from build123d import *

# Parameters (mm, degrees)
SKETCH21_R          = 1.625
SKETCH21_R_2        = 7.5
MAIN_DEPTH          = 2
SKETCH23_R          = 4.2
SKETCH23_R_2        = 3.2
BOSS_EXTRUDE1_DEPTH = 2
REVOLVE1_START      = 2
REVOLVE1_DEPTH      = 3.0000001
REVOLVE1_2_ANGLE    = 20
REVOLVE1_3_ANGLE    = 20
CIRPATTERN1_COUNT   = 4


with BuildPart() as part:
    # Sketch21 → Main (new body)
    with BuildSketch(Plane(origin=(0, 0, 0), x_dir=(1, 0, 0), z_dir=(0, 1, 0))):
        with BuildLine():
            Line((-12.374368671, 10.960155108), (-10.960155108, 12.374368671))
            ThreePointArc((-10.960155108, 12.374368671), (-8.838834765, 13.253048327), (-6.717514421, 12.374368671))
            Line((-6.717514421, 12.374368671), (-6.969531846, 12.626386096))
            ThreePointArc((-6.969531846, 12.626386096), (-5.176380902, 11.591109915), (-3.105828541, 11.591109915))
            ThreePointArc((-3.105828541, 11.591109915), (0, 12), (3.105828541, 11.591109915))
            ThreePointArc((3.105828541, 11.591109915), (5.176380902, 11.591109915), (6.969531846, 12.626386096))
            Line((6.969531846, 12.626386096), (6.717514421, 12.374368671))
            ThreePointArc((6.717514421, 12.374368671), (8.838834765, 13.253048327), (10.960155108, 12.374368671))
            Line((10.960155108, 12.374368671), (12.374368671, 10.960155108))
            ThreePointArc((12.374368671, 10.960155108), (13.253048327, 8.838834765), (12.374368671, 6.717514421))
            Line((12.374368671, 6.717514421), (12.626386096, 6.969531846))
            ThreePointArc((12.626386096, 6.969531846), (11.591109915, 5.176380902), (11.591109915, 3.105828541))
            ThreePointArc((11.591109915, 3.105828541), (12, 0), (11.591109915, -3.105828541))
            ThreePointArc((11.591109915, -3.105828541), (11.591109915, -5.176380902), (12.626386096, -6.969531846))
            Line((12.626386096, -6.969531846), (12.374368671, -6.717514421))
            ThreePointArc((12.374368671, -6.717514421), (13.253048327, -8.838834765), (12.374368671, -10.960155108))
            Line((12.374368671, -10.960155108), (10.960155108, -12.374368671))
            ThreePointArc((10.960155108, -12.374368671), (8.838834765, -13.253048327), (6.717514421, -12.374368671))
            Line((6.717514421, -12.374368671), (6.969531846, -12.626386096))
            ThreePointArc((6.969531846, -12.626386096), (5.176380902, -11.591109915), (3.105828541, -11.591109915))
            ThreePointArc((3.105828541, -11.591109915), (0, -12), (-3.105828541, -11.591109915))
            ThreePointArc((-3.105828541, -11.591109915), (-5.176380902, -11.591109915), (-6.969531846, -12.626386096))
            Line((-6.969531846, -12.626386096), (-6.717514421, -12.374368671))
            ThreePointArc((-6.717514421, -12.374368671), (-8.838834765, -13.253048327), (-10.960155108, -12.374368671))
            Line((-10.960155108, -12.374368671), (-12.374368671, -10.960155108))
            ThreePointArc((-12.374368671, -10.960155108), (-13.253048327, -8.838834765), (-12.374368671, -6.717514421))
            Line((-12.374368671, -6.717514421), (-12.626386096, -6.969531846))
            ThreePointArc((-12.626386096, -6.969531846), (-11.591109915, -5.176380902), (-11.591109915, -3.105828541))
            ThreePointArc((-11.591109915, -3.105828541), (-12, 0), (-11.591109915, 3.105828541))
            ThreePointArc((-11.591109915, 3.105828541), (-11.591109915, 5.176380902), (-12.626386096, 6.969531846))
            Line((-12.626386096, 6.969531846), (-12.374368671, 6.717514421))
            ThreePointArc((-12.374368671, 6.717514421), (-13.253048327, 8.838834765), (-12.374368671, 10.960155108))
        make_face()
        with Locations(Location((8.838834765, 8.838834765, 0), (0, 0, 270))):
            Circle(SKETCH21_R, mode=Mode.SUBTRACT)
        with Locations(Location((8.838834765, -8.838834765, 0), (0, 0, 270))):
            Circle(SKETCH21_R, mode=Mode.SUBTRACT)
        with Locations(Location((-8.838834765, -8.838834765, 0), (0, 0, 270))):
            Circle(SKETCH21_R, mode=Mode.SUBTRACT)
        with Locations(Location((-8.838834765, 8.838834765, 0), (0, 0, 270))):
            Circle(SKETCH21_R, mode=Mode.SUBTRACT)
        with Locations(Location((0, 0, 0), (0, 0, 270))):
            Circle(SKETCH21_R_2, mode=Mode.SUBTRACT)
    extrude(amount=MAIN_DEPTH)



with BuildPart() as body_2:
    # Sketch23 → Boss-Extrude1 (new body)
    with BuildSketch(Plane(origin=(0, 5, 0), x_dir=(1, 0, 0), z_dir=(0, 1, 0))):
        with Locations(Location((0, 0, 0), (0, 0, 270))):
            Circle(SKETCH23_R)
        with Locations(Location((0, 0, 0), (0, 0, 270))):
            Circle(SKETCH23_R_2, mode=Mode.SUBTRACT)
    extrude(amount=-BOSS_EXTRUDE1_DEPTH)


with BuildPart() as part_1:
    add(part.part)

    add(body_2.part)  # Revolve1 merges body 2
    # Revolve1: read off the stored shape, not the designer's step
    # Revolve1 outline → Revolve1 (add)
    with BuildSketch(Plane(origin=(0, 0, 0), x_dir=(1, 0, 0), z_dir=(0, 1, 0)).offset(REVOLVE1_START)):
        with BuildLine():
            ThreePointArc((-7.386058148, 1.302361332), (-7.5, 0), (-7.386058148, -1.302361332))
            Line((-7.386058148, -1.302361332), (-4.136192563, -0.729322346))
            ThreePointArc((-4.136192563, -0.729322346), (-4.2, 0), (-4.136192563, 0.729322346))
            Line((-4.136192563, 0.729322346), (-7.386058148, 1.302361332))
        make_face()
    revolve1 = extrude(amount=REVOLVE1_DEPTH)

    # Revolve1 2 outline → Revolve1 2 (revolve, cut)
    with BuildSketch(Plane(origin=(0, 0, 0), x_dir=(-0.9848077530122078, 0, -0.17364817766693202), z_dir=(0.17364817766693202, 0, -0.9848077530122078))):
        with BuildLine():
            Line((7.5, 5.0000001), (4.2, 5))
            add(Edge.make_bspline(
                [(4.2, 5), (5.982635205, 4.992310164), (6.774082879, 4.851938269), (7.492555324, 4.584836693), (7.5, 4.582052306)],
                knots=[0, 0, 0, 0, 0.380988924, 0.384982373, 0.384982373, 0.384982373, 0.384982373], degree=3))
            Line((7.5, 4.582052306), (7.5, 5.0000001))
        make_face()
        with BuildLine():
            Line((5.505892852, 3), (4.2, 3))
            Line((4.2, 3), (4.2, 2))
            Line((4.2, 2), (7.5, 2))
            Line((7.5, 2), (7.5, 2.168694052))
            add(Edge.make_bspline(
                [(7.5, 2.168694052), (7.474165676, 2.402361508), (7.259227976, 2.776784864), (6.698722273, 2.938737477), (6.279860406, 2.965955752), (5.872473083, 2.987273734), (5.643353064, 2.995990887), (5.505892852, 3)],
                knots=[0.04346167, 0.04346167, 0.04346167, 0.04346167, 0.224146676, 0.342653564, 0.481775745, 0.553286067, 0.660507352, 0.660507352, 0.660507352, 0.660507352], degree=3))
        make_face()
        with BuildLine():
            add(Edge.make_bspline(
                [(5.505892852, 3), (5.070655283, 3.012693977), (4.635308795, 3.013153878), (4.2, 3)],
                knots=[0.660507352, 0.660507352, 0.660507352, 0.660507352, 1, 1, 1, 1], degree=3))
            Line((4.2, 3), (5.505892852, 3))
        make_face()
    revolve1_2 = revolve(axis=Axis((0, 0, 0), (0, 1, 0)), revolution_arc=REVOLVE1_2_ANGLE, mode=Mode.SUBTRACT)

    # Revolve1 3 outline → Revolve1 3 (revolve)
    with BuildSketch(Plane(origin=(0, 0, 0), x_dir=(-0.9848077530122078, 0, -0.17364817766693202), z_dir=(0.17364817766693202, 0, -0.9848077530122078))):
        with BuildLine():
            Line((7.5, 4.582052306), (7.5, 2.168694052))
            add(Edge.make_bspline(
                [(7.5, 2), (7.506412796, 2.055845291), (7.506214145, 2.112488071), (7.5, 2.168694052)],
                knots=[0, 0, 0, 0, 0.04346167, 0.04346167, 0.04346167, 0.04346167], degree=3))
            Line((7.5, 2), (9.5, 2))
            add(Edge.make_bspline(
                [(9.5, 2), (9.601210283, 3.398928444), (8.64652948, 4.15323827), (7.5, 4.582052306)],
                knots=[0.969922529, 0.969922529, 0.969922529, 0.969922529, 1.584940156, 1.584940156, 1.584940156, 1.584940156], degree=3))
        make_face()
    revolve1_3 = revolve(axis=Axis((0, 0, 0), (0, 1, 0)), revolution_arc=REVOLVE1_3_ANGLE)

    # CirPattern1: Revolve1, Revolve1 2, Revolve1 3 ×4 about axis
    cirpattern1_axis = Axis((0, -52.54930657, 0), (0, 1, 0))
    add([revolve1.rotate(cirpattern1_axis, i * 360 / CIRPATTERN1_COUNT) for i in range(1, CIRPATTERN1_COUNT)])
    add([revolve1_2.rotate(cirpattern1_axis, i * 360 / CIRPATTERN1_COUNT) for i in range(1, CIRPATTERN1_COUNT)], mode=Mode.SUBTRACT)
    add([revolve1_3.rotate(cirpattern1_axis, i * 360 / CIRPATTERN1_COUNT) for i in range(1, CIRPATTERN1_COUNT)])


solid = part_1.part
Geometry check sheet. Reference: the model listing, model coordinates, mm. A direction names the side the tool comes from. Coordinates: 2 decimals unless noted, no trailing zeros. Order: outer loops, then holes, each group sorted by start corner. A loop starts at its lowest first (then second) coordinate and runs counter-clockwise, first axis right, second up. Notation, with made-up numbers: (10.25, -37) - (54.25, -37) arc R20 cw to (54.25, 0) - close; hole circle Ø5 at (-13, 17.5). An arc over 180 degrees is marked (long way). Answer in a Markdown table with one row per item. Add a question column.
1) Release check for a two-part mould opening along Z. For faces 5 (the flat face through (-11.677, 0.986, -11.657)), 6 (the cylindrical face through (9.937, 0.986, 7.641)), 7 (the cylindrical face through (0, 1, 12)) record: +Z half, -Z half, draft (parallel to the pull), parting line (faces both ways), or undercut.
2) Cross-section at B-B, the plane y = 0.4. State how many separate pieces and enclosed holes the cut face has, then the cut area to 3 significant figures.
3) Set-up check for faces 1 (the flat face through (-6, 2, 6)), 2 (the cylindrical face through (-2.94, 4.01, -3)), 3 (the flat face through (-2, 3, -3)), 4 (the cylindrical face through (-11.599, 0.986, 5.205)): record each of +Z, -Z, +X, -X, +Y, -Y from which the full face is reachable in a straight line by a thin tool's end or side.
4) Cross-section at C-C, the plane z = 2. Record the cut outline in (x, y).
5) Material ranges on line 1 along Z through (x, y) = (10, 1.1); line 2 along Y through (x, z) = (-7.5, 2.75); line 3 along X through (y, z) = (0.65, 4.5), recorded low to high. Write a range as [from, to].
6) Gauge pin test, flat ends, axial feed: P1, Ø1.9, axis at x = 8.84, z = -8.84, coming from the -Y side; P2, Ø1.5, axis at y = 0.5, z = 5.5, coming from the -X side; P3, Ø1.5, axis at x = 2.5, y = 2.5, coming from the +Z side; P4, Ø2, axis at x = -5.5, z = -5.5, coming from the +Y side. Record the tip position at first contact, or that the pin passes through.
7) Cross-section at A-A, the plane z = -2.25. Record the cut outline in (x, y), then the cut area to 3 significant figures.
Check result:
| question | item | result |
|---|---|---|
| 1 | face 5 | -Z half |
| 1 | face 6 | undercut |
| 1 | face 7 | +Z half |
| 2 | separate pieces | 1 |
| 2 | enclosed holes | 5 |
| 2 | area | 386 mm² |
| 3 | face 1 | +Y |
| 3 | face 2 | +Y, -Y |
| 3 | face 3 | -Y |
| 3 | face 4 | -X, +Y, -Y |
| 4 | outline | (-11.83, 0) - (-7.23, 0) - (-7.23, 2) - (-11.83, 2) - close; (-3.69, 3) - (-2.5, 3) - (-2.5, 5) - (-3.69, 5) - close; (2.5, 3) - (3.69, 3) - (3.69, 5) - (2.5, 5) - close; (7.23, 0) - (11.83, 0) - (11.83, 2) - (7.23, 2) - close |
| 5 | line 1 | z = [-13.02, -9.98], [-7.7, 7.7], [9.98, 13.02] |
| 5 | line 2 | y = [0, 2] |
| 5 | line 3 | x = [-11.47, -6], [6, 11.47] |
| 6 | P1 | passes through |
| 6 | P2 | stops at x = -12.06 |
| 6 | P3 | stops at z = 11.84 |
| 6 | P4 | stops at y = 2 |
| 7 | outline | (-11.79, 0) - (-7.15, 0) - (-7.15, 2) - (-11.79, 2) - close; (-3.55, 3) - (-2.28, 3) - (-2.28, 5) - (-3.55, 5) - close; (2.28, 3) - (3.55, 3) - (3.55, 5) - (2.28, 5) - close; (7.15, 0) - (11.79, 0) - (11.79, 2) - (7.15, 2) - close |
| 7 | area | 23.6 mm² |
